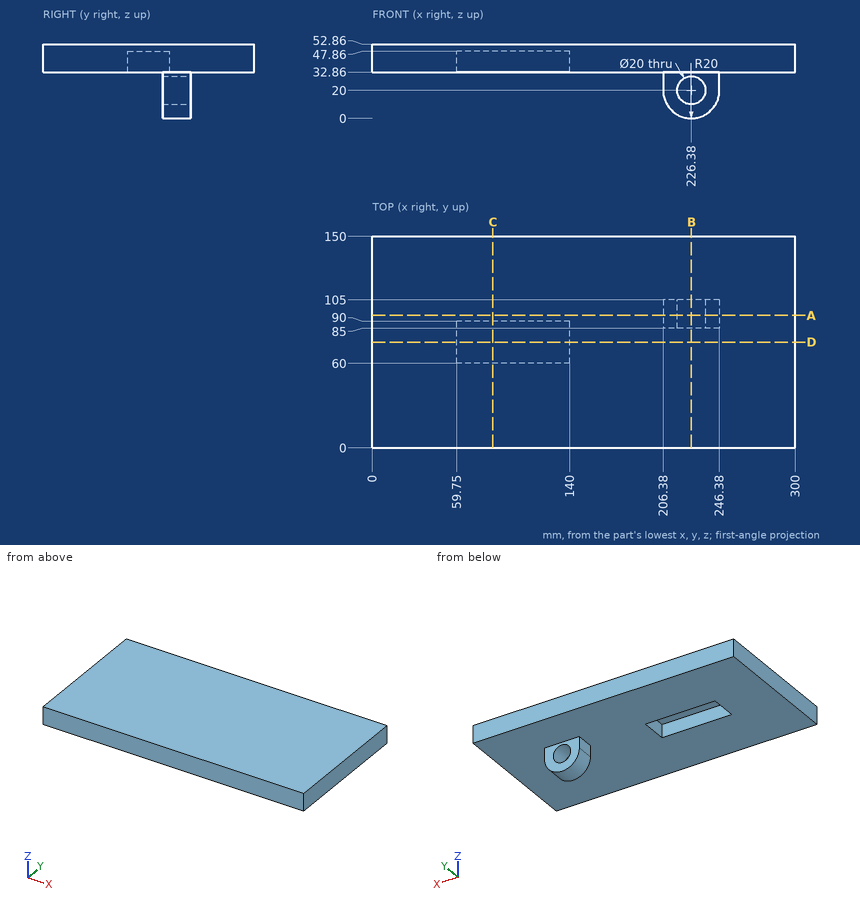
Design review of the part shown in the three views and the two pictorial views. Dimensions are in mm from the part's minimum x, y and z. Coordinates: 2 decimals unless noted, no trailing zeros. Write each loop counter-clockwise with the first axis right and the second up, starting at its lowest first coordinate (ties: lowest second). Pieces come first, ordered by that corner, then holes. Notation, with made-up numbers: (-11, -19.75) - (-1, -19.75) arc R10 ccw to (-1, -0.75) - close; hole circle Ø11 at (-29, 81). An arc over 180 degrees is marked (long way). Write item = value, one per line.
(1) Consider section B-B, the plane x = 226.38. Give the boundary of the cut face in (y, z).
Result sheet:
outline = (0, 32.86) - (85, 32.86) - (85, 30) - (105, 30) - (105, 32.86) - (150, 32.86) - (150, 52.86) - (0, 52.86) - close; (85, 0) - (105, 0) - (105, 10) - (85, 10) - close
(2) Consider section D-D, the plane y = 75. Give the boundary of the cut face in (x, z), then the cut area to 3 significant figures.
Result sheet:
outline = (0, 32.86) - (59.75, 32.86) - (59.75, 47.86) - (140, 47.86) - (140, 32.86) - (300, 32.86) - (300, 52.86) - (0, 52.86) - close
area = 4,800 mm^2
(3) For line 1 (Z direction, x = 226.38, y = 98.75); line 2 (X direction, y = 90, z = 20); line 3 (Z direction, x = 115, y = 110.5), list the stretches that pass through material, from the lowest coordinate up. Write a range as [from, to].
Result sheet:
line_1 = [0, 10], [30, 52.86]
line_2 = [206.38, 216.38], [236.38, 246.38]
line_3 = [32.86, 52.86]
(4) Consider section A-A, the plane y = 94. Give the boundary of the cut face in (x, z), then the cut area to 3 significant figures.
Result sheet:
outline = (0, 32.86) - (206.38, 32.86) - (206.38, 20) arc R20 ccw to (246.38, 20) - (246.38, 32.86) - (300, 32.86) - (300, 52.86) - (0, 52.86) - close; hole circle Ø20 at (226.38, 20)
area = 6,830 mm^2
(5) Consider section C-C, the plane x = 85.5. Give the boundary of the cut face in (y, z), then the cut area to 3 significant figures.
Result sheet:
outline = (0, 32.86) - (60, 32.86) - (60, 47.86) - (90, 47.86) - (90, 32.86) - (150, 32.86) - (150, 52.86) - (0, 52.86) - close
area = 2,550 mm^2
(6) For P1, Ø1, axis at x = 229.5, y = 65.5, coming from the -Z side; P2, Ø6.5, axis at y = 91, z = 24.5, coming from the +X side; P3, Ø15, axis at x = 86.5, y = 74.5, coming from the -Z side, all flat-tipped, find the tip position at first contact; note any pin that passes through.
Result sheet:
P1 = 32.86
P2 = 246.38
P3 = 47.86
